from build123d import *

# Parameters (mm, degrees)
F0_W     = 76.2
F0_H     = 63.5
F1_DEPTH = 38.1
F2_W     = 76.2
F2_H     = 19.05
F7_DEPTH = 127
F4_D     = 19.84248
F6_DEPTH = 38.1


with BuildPart() as f1:
    # F0 (on Top) → F1 (new body)
    with BuildSketch(Plane.XY):
        Rectangle(F0_W, F0_H)
    extrude(amount=F1_DEPTH)

    # F2 (on face) → F7 (join)
    with BuildSketch(Plane.XY.offset(38.1)):
        with Locations((0, 22.225)):
            Rectangle(F2_W, F2_H)
    extrude(amount=F7_DEPTH)

    # F4 (through all)
    with Locations(Plane(origin=(0, 31.75, 0), x_dir=(-1, 0, 0), z_dir=(0, 1, 0))):
        with Locations((0, 63.2342693158)):
            Hole(F4_D / 2)

    # F5 (on face) → F6 (cut, through all)
    with BuildSketch(Plane.XZ.offset(31.75)):
        with BuildLine():
            Line((38.1, 38.1), (-38.1, 38.1))
            ThreePointArc((-38.1, 38.1), (0, 31.7262437458), (38.1, 38.1))
        make_face()
    extrude(amount=-F6_DEPTH, mode=Mode.SUBTRACT)


solid = f1.part
The listing builds one solid part. Answer for the finished solid, in the listing's coordinates (mm). A direction names the side the tool comes from. Coordinates: 2 decimals unless noted, no trailing zeros. Loops run counter-clockwise (first coordinate to the right, second up) from the corner with the lowest first, then second, coordinate; pieces in that order, holes last. Notation, with made-up numbers: M -18.75,77 L 9.25,77 A16 ccw 9.25,88 Z; hole C 23.5,0.25 d6. An arc over 180 degrees is marked long. Answer in a Markdown table with one row per item.
1) Determine the mould class of faces 4 (the flat face through (-1, 6.35, 36)), 5 (the flat face through (-1, 22, 165.1)), 6 (the cylindrical face through (-1.29, 22.09, 73.07)) for opening direction Z: released by +Z, released by -Z, zero draft, split by the parting line, or undercut.
Answers below:
| item | result |
|---|---|
| face 4 | zero draft |
| face 5 | released by +Z |
| face 6 | undercut |
2) Given pin 1 (1.9 mm diameter, centred on x = 9.5, y = 8, fed in from +Z); pin 2 (23 mm diameter, centred on x = 0, z = 63.23, fed in from -Y); pin 3 (1.9 mm diameter, centred on x = -3.5, z = 34, fed in from -Y), each flat-ended and moving along its own axis, determine where each tip first touches the part or whether it passes through.
Answers below:
| item | result |
|---|---|
| pin 1 | z = 38.1 |
| pin 2 | y = 12.7 |
| pin 3 | y = 6.35 |
3) Find section C-C (x = 19.5). Determine the outline of the cut face in (y, z).
Answers below:
| item | result |
|---|---|
| outline | M -31.75,0 L 31.75,0 L 31.75,165.1 L 12.7,165.1 L 12.7,38.1 L 6.35,38.1 L 6.35,33.36 L -31.75,33.36 Z |
4) Find section B-B (z = 58). Determine the outline of the cut face in (x, y).
Answers below:
| item | result |
|---|---|
| outline | M -38.1,12.7 L -8.43,12.7 L -8.43,31.75 L -38.1,31.75 Z; M 8.43,12.7 L 38.1,12.7 L 38.1,31.75 L 8.43,31.75 Z |
5) Find the intervals of material crossed by probe 1 along Z at (x, y) = (0, 27); probe 2 along Y at (x, z) = (-15, 70.5); probe 3 along Z at (x, y) = (3, 16.5), in increasing order.
Answers below:
| item | result |
|---|---|
| probe 1 | 0 to 53.31, 73.16 to 165.1 |
| probe 2 | 12.7 to 31.75 |
| probe 3 | 0 to 53.78, 72.69 to 165.1 |
6) Which of the six approach directions +Z, -Z, +X, -X, +Y, -Y give full straight-line access (tool end or side, diameter ignored) to faces 1 (the flat face through (-1, 12.7, 101)), 2 (the cylindrical face through (-0.543, -12.967, 31.728)), 3 (the flat face through (-38.1, 14, 63))?
Answers below:
| item | result |
|---|---|
| face 1 | +Z, +X, -X, -Y |
| face 2 | +Z, -Y |
| face 3 | +Z, -Z, -X, +Y, -Y |
7) Find section D-D (y = 24.5). Determine the outline of the cut face in (x, z), then the cut area to 3 significant figures.
Answers below:
| item | result |
|---|---|
| outline | M -38.1,0 L 38.1,0 L 38.1,165.1 L -38.1,165.1 Z; hole C 0,63.23 d19.84 |
| area | 12,300 mm^2 |
8) Find section A-A (x = 0). Determine the outline of the cut face in (y, z), then the cut area to 3 significant figures.
Answers below:
| item | result |
|---|---|
| outline | M -31.75,0 L 31.75,0 L 31.75,53.31 L 12.7,53.31 L 12.7,38.1 L 6.35,38.1 L 6.35,31.73 L -31.75,31.73 Z; M 12.7,73.16 L 31.75,73.16 L 31.75,165.1 L 12.7,165.1 Z |
| area | 4,220 mm^2 |
